For this review, use the dimensioned drawing (mm, ordinates from the lowest corner) and the shaded views. Coordinates: 2 decimals unless noted, no trailing zeros. Loops run counter-clockwise (first coordinate to the right, second up) from the corner with the lowest first, then second, coordinate; pieces in that order, holes last. Notation, with made-up numbers: (17.5, 60.25) - (31.5, 60.25) arc R35 ccw to (31.5, 95.25) - close; hole circle Ø5 at (66, -32). An arc over 180 degrees is marked (long way). Answer in a Markdown table with one row per item. Add a question column.
(1) We need section C-C, the plane x = 7. Write out the cut boundary in (y, z), plus the area to 3 significant figures.
(2) We need section B-B, the plane z = 49. Write out the cut boundary in (x, y).
(3) Clearance check with flat-ended pins moving along their axes: pin 1 (12 mm diameter, centred on x = 87, z = 28, fed in from -Y); pin 2 (8 mm diameter, centred on x = 93, y = 20, fed in from -Z); pin 3 (2 mm diameter, centred on x = 79.5, y = 31.5, fed in from -Z); pin 4 (5.5 mm diameter, centred on x = 7, y = 20, fed in from -Z) (1 decimal). State where each tip first meets the part, or that it passes through.
(4) We need section A-A, the plane y = 20. Write out the cut boundary in (x, z), plus the area to 3 significant figures.
(5) We need section D-D, the plane x = 42.5. Write out the cut boundary in (y, z), plus the area to 3 significant figures.
(6) To check wall thickness, follow L1, parallel to Y at x = 93, z = 28; L2, parallel to X at y = 21.5, z = 41.5; L3, parallel to Z at x = 90, y = 22. State the ranges of each line that lie inside material, in increasing order. Write a range as [from, to].
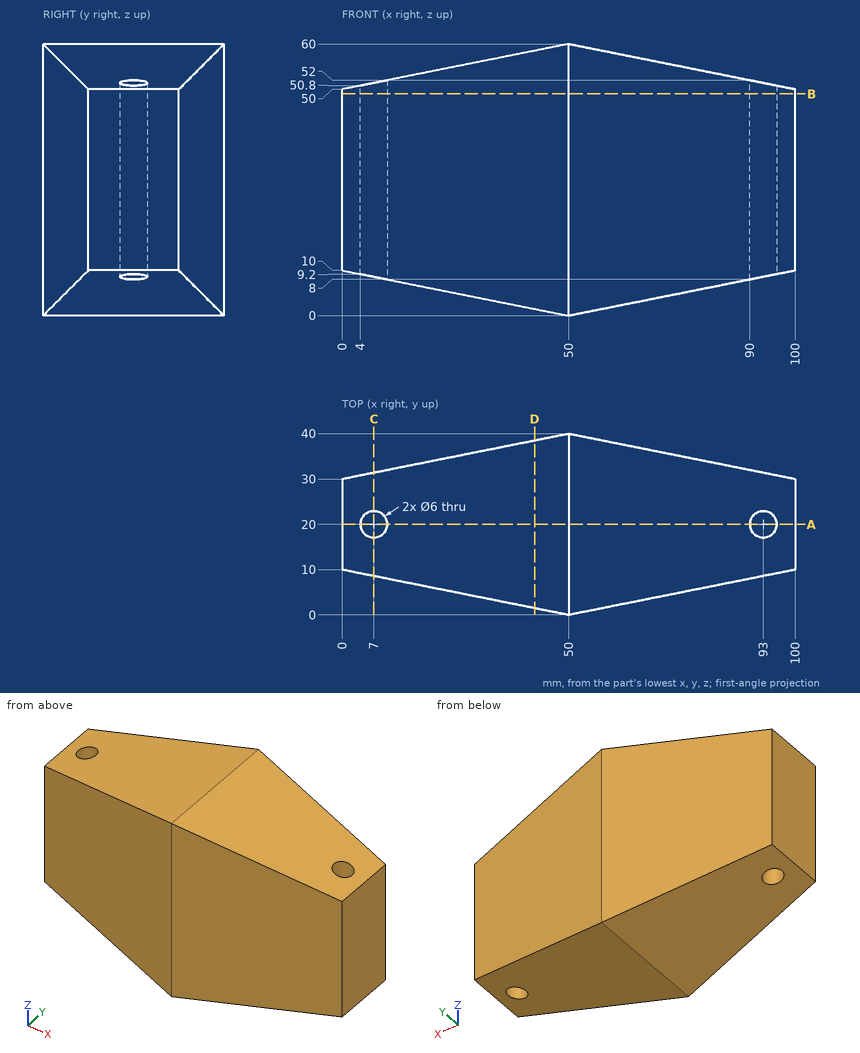
Responses:
| question | item | result |
|---|---|---|
| 1 | outline | (8.6, 8.6) - (17, 8.6) - (17, 51.4) - (8.6, 51.4) - close; (23, 8.6) - (31.4, 8.6) - (31.4, 51.4) - (23, 51.4) - close |
| 1 | area | 719 mm2 |
| 2 | outline | (0, 10) - (50, 0) - (100, 10) - (100, 30) - (50, 40) - (0, 30) - close; hole circle Ø6 at (7, 20); hole circle Ø6 at (93, 20) |
| 3 | pin 1 | stops at y = 6.2 |
| 3 | pin 2 | stops at z = 7.8 |
| 3 | pin 3 | stops at z = 5.7 |
| 3 | pin 4 | passes through |
| 4 | outline | (0, 10) - (4, 9.2) - (4, 50.8) - (0, 50) - close; (10, 8) - (50, 0) - (90, 8) - (90, 52) - (50, 60) - (10, 52) - close; (96, 9.2) - (100, 10) - (100, 50) - (96, 50.8) - close |
| 4 | area | 4,490 mm2 |
| 5 | outline | (1.5, 1.5) - (38.5, 1.5) - (38.5, 58.5) - (1.5, 58.5) - close |
| 5 | area | 2,110 mm2 |
| 6 | L1 | y = [8.6, 17], [23, 31.4] |
| 6 | L2 | x = [0, 4.4], [9.6, 90.4], [95.6, 100] |
| 6 | L3 | z = [8, 52] |
